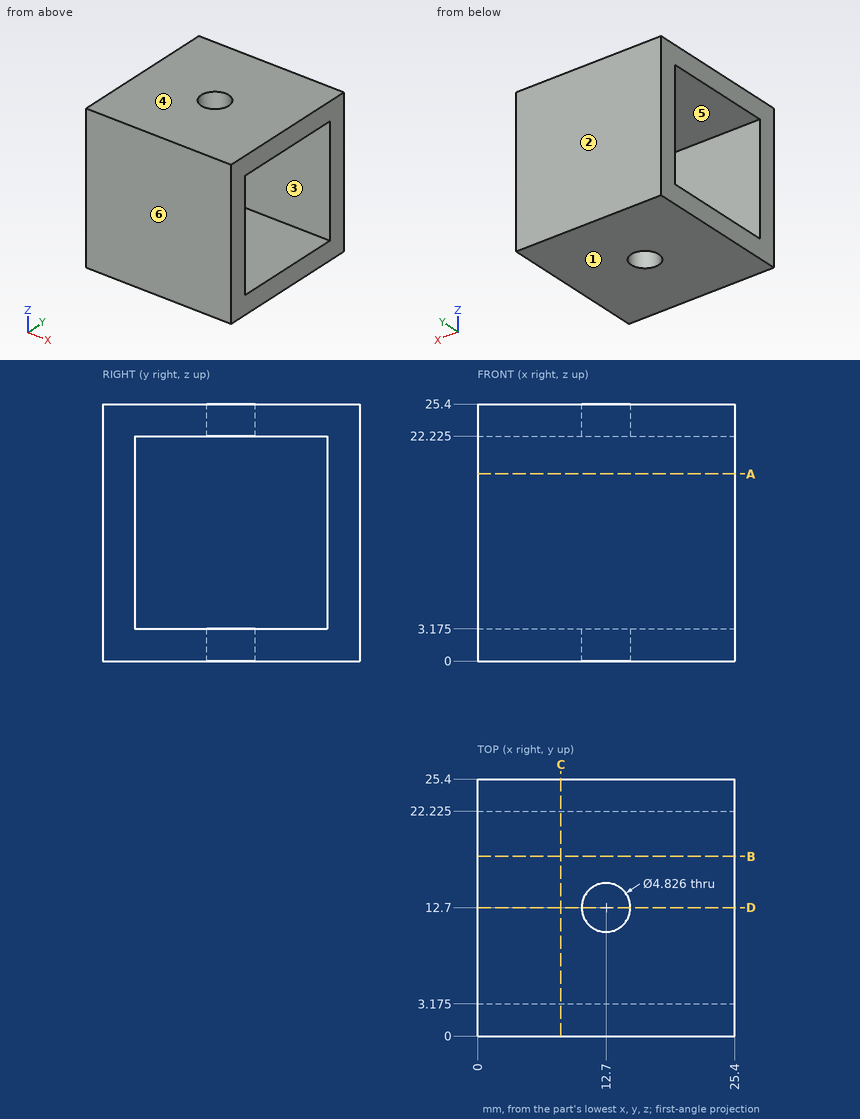
Job drawing, mm, ordinate dimensions from the low corner. One solid piece. A direction names the side the tool comes from. Give positions to 0.01 mm unless a question says otherwise; leave off trailing zeros. Loops run counter-clockwise (first coordinate to the right, second up) from the corner with the lowest first, then second, coordinate; pieces in that order, holes last. Notation, with made-up numbers: (14, -26.75) -> (61, -26.75) arc R19 cw to (61, 5.25) -> close; hole circle Ø8 at (-13, 51). An arc over 180 degrees is marked (long way). Write each question's results on one line, items separated by ' | '.
(1) Tool access for the marked faces 5 and 6: list every direction of +Z, -Z, +X, -X, +Y, -Y with a clear straight run to the whole face (end or side of a thin tool).
Geometry results:
face 5: +X, -X | face 6: +Z, -Z, +X, -X, -Y
(2) Cut at A-A on z = 18.5. List the corners of the cut face in (x, y) (3 decimals).
Geometry results:
outline: (0, 0) -> (25.4, 0) -> (25.4, 3.175) -> (0, 3.175) -> close; (0, 22.225) -> (25.4, 22.225) -> (25.4, 25.4) -> (0, 25.4) -> close
(3) Probe line 1 along Z through (x, y) = (15.5, 3.5) (3 decimals); line 2 along Y through (x, z) = (12.7, 2.25). List the from-to ranges inside material, lowest first.
Geometry results:
line 1: z = 0 to 3.175, 22.225 to 25.4 | line 2: y = 0 to 10.29, 15.11 to 25.4
(4) Pull direction Z, two halves, no side cores. Call the marked faces 1, 2, 3 and 4: released by +Z, released by -Z, zero draft, split by the parting line, or undercut.
Geometry results:
face 1: released by -Z | face 2: zero draft | face 3: undercut | face 4: released by +Z
(5) Cut at C-C on x = 8.25. List the corners of the cut face in (y, z) (3 decimals), and give its area (3 significant figures).
Geometry results:
outline: (0, 0) -> (25.4, 0) -> (25.4, 25.4) -> (0, 25.4) -> close; hole (3.175, 3.175) -> (22.225, 3.175) -> (22.225, 22.225) -> (3.175, 22.225) -> close | area: 282 mm²
(6) Cut at D-D on y = 12.7. List the corners of the cut face in (x, z) (3 decimals), and give its area (3 significant figures).
Geometry results:
outline: (0, 0) -> (10.287, 0) -> (10.287, 3.175) -> (0, 3.175) -> close; (0, 22.225) -> (10.287, 22.225) -> (10.287, 25.4) -> (0, 25.4) -> close; (15.113, 0) -> (25.4, 0) -> (25.4, 3.175) -> (15.113, 3.175) -> close; (15.113, 22.225) -> (25.4, 22.225) -> (25.4, 25.4) -> (15.113, 25.4) -> close | area: 131 mm²
